Check sheet for the modelled part. Datum: model origin and axes. Units: mm. A direction names the side the tool comes from. Give positions to 0.01 mm unless a question says otherwise; leave off trailing zeros. Loops run counter-clockwise (first coordinate to the right, second up) from the corner with the lowest first, then second, coordinate; pieces in that order, holes last. Notation, with made-up numbers: M 78.5,-11 L 104.5,-11 A8 cw 104.5,-4 Z; hole C -1.5,17.25 d3. An arc over 180 degrees is marked long. Write each question's results on one line, items separated by ' | '. Start each with the question number.
1. Sectioned sample at A-A on z = 3.25. Record the cut outline in (x, y).
2. Sectioned sample at C-C on y = -7.5. Record the cut outline in (x, z).
3. Sectioned sample at D-D on x = -13.5. Record the cut outline in (y, z), and give its area (3 significant figures).
4. Tool access check on faces 1 (the flat face through (-17.1, 4, 3)), 2 (the flat face through (-16.6, -6, 1)), 3 (the flat face through (19, 2.9, 13)). Record the directions out of +Z, -Z, +X, -X, +Y, -Y that give a thin tool (end or side, any length) a straight path to the whole face; none if there is none.
5. Material ranges on line 1 along Z through (x, y) = (10, -5.75); line 2 along X through (y, z) = (5, 20), recorded low to high.
6. Sectioned sample at B-B on z = 21.25. Record the cut outline in (x, y), and give its area (3 significant figures).
7. Draft check along Y on faces 4 (the flat face through (19.6, 5.8, 24)), 5 (the flat face through (-19.1, 6, 3)), 6 (the flat face through (-19, 2.9, 3)), 7 (the flat face through (19.1, 6, 13)). Enter one of: pulls with the +Y half, pulls with the -Y half, needs draft (parallel to the pull), parting line crosses it, or undercut.
8. Go/stop test with flat-tipped pins: pin 1 (0.6 mm diameter, centred on y = 7.5, z = 8.5, fed in from -X); pin 2 (1 mm diameter, centred on x = 18, z = 16, fed in from -Y); pin 3 (6 mm diameter, centred on x = -6.5, y = 6.5, fed in from +Z). Record where each tip stops, or that it passes through.
Autodesk Inventor part; units mm, degrees
ref_plane "YZ Plane" through (0, 0, 0) normal (1, 0, 0) x (0, 1, 0)
ref_plane "XZ Plane" through (0, 0, 0) normal (0, 1, 0) x (-1, 0, 0)
ref_plane "XY Plane" through (0, 0, 0) normal (0, 0, 1) x (1, 0, 0)
sketch "Sketch1" plane through (0, 0, 0) normal (0, 0, 1) x (1, 0, 0)
  line L0 (20.1, 8.7) -> (-20.1, 8.7)
  line L1 (-20.1, 8.7) -> (-20.1, -8.7)
  line L2 (-20.1, -8.7) -> (20.1, -8.7)
  line L3 (20.1, -8.7) -> (20.1, 8.7)
  line L4 (20.1, 8.7) -> (-20.1, -8.7) construction
  line L5 (-20.1, 8.7) -> (20.1, -8.7) construction
  line L6 (-20.1, -8.7) -> (-16.6, -8.7)
  line L7 (-16.6, -8.7) -> (-16.6, -3.5)
  line L8 (-16.6, -3.5) -> (-20.1, -3.5)
  line L9 (-20.1, -3.5) -> (-20.1, -8.7)
  point P0 (0, 0)
  point P1 (-16.6, -8.7)
  dimension "d0" = 40.2
  dimension "d1" = 17.4
  dimension "d3" = 5.2
  dimension "d20" = 36.7
extrude "Extrusion1" add sketch "Sketch1" along normal blind 2 contours L3 L2 L7 L8 L1 L0
sketch "Sketch2" plane through (0, 0, 2) normal (0, 0, 1) x (1, 0, 0)
  line L0 (-20.1, 8.7) -> (-20.1, -3.5)
  line L1 (-20.1, 8.7) -> (-17.1, 8.7)
  line L2 (-17.1, 8.7) -> (-17.1, 2.9)
  line L3 (-17.1, 2.9) -> (-20.1, 2.9)
  line L4 (-20.1, 2.9) -> (-20.1, 8.7)
  line L5 (20.1, -8.7) -> (20.1, 8.7)
  line L6 (20.1, 8.7) -> (17.1, 8.7)
  line L7 (17.1, 8.7) -> (17.1, 2.9)
  line L8 (17.1, 2.9) -> (20.1, 2.9)
  line L9 (20.1, 2.9) -> (20.1, 8.7)
  line L10 (-20.1, 2.9) -> (-17.1, 2.9)
  line L11 (-17.1, 2.9) -> (-17.1, 4.9)
  line L12 (-17.1, 4.9) -> (-20.1, 4.9)
  line L13 (-20.1, 4.9) -> (-20.1, 2.9)
  line L14 (-20.1, 8.7) -> (-17.1, 8.7)
  line L15 (-17.1, 8.7) -> (-17.1, 6.7)
  line L16 (-17.1, 6.7) -> (-20.1, 6.7)
  line L17 (-20.1, 6.7) -> (-20.1, 8.7)
  line L18 (-20.1, 6.7) -> (-19.1, 6.7)
  line L19 (-19.1, 6.7) -> (-19.1, 4.9)
  line L20 (-19.1, 4.9) -> (-20.1, 4.9)
  line L21 (-20.1, 4.9) -> (-20.1, 6.7)
  line L22 (20.1, 8.7) -> (17.1, 8.7)
  line L23 (17.1, 8.7) -> (17.1, 6.7)
  line L24 (17.1, 6.7) -> (20.1, 6.7)
  line L25 (20.1, 6.7) -> (20.1, 8.7)
  line L26 (17.1, 2.9) -> (20.1, 2.9)
  line L27 (20.1, 2.9) -> (20.1, 4.9)
  line L28 (20.1, 4.9) -> (17.1, 4.9)
  line L29 (17.1, 4.9) -> (17.1, 2.9)
  line L30 (20.1, 4.9) -> (19.1, 4.9)
  line L31 (19.1, 4.9) -> (19.1, 6.7)
  line L32 (19.1, 6.7) -> (20.1, 6.7)
  line L33 (20.1, 6.7) -> (20.1, 4.9)
  point P0 (0, 0)
  dimension "d6" = 3
  dimension "d7" = 5.8
  dimension "d8" = 3
  dimension "d9" = 5.8
  dimension "d10" = 2
  dimension "d11" = 2
  dimension "d12" = 1
  dimension "d13" = 2
  dimension "d14" = 2
  dimension "d15" = 1
extrude "Extrusion2" add sketch "Sketch2" along normal blind 3 contours L1 L2 L16 L0 | L16 L19 L12 L0 | L12 L2 L3 L0 | L8 L7 L28 L5 | L28 L31 L24 L5 | L24 L7 L6 L5
sketch "Sketch3" plane through (0, 0, 5) normal (0, 0, 1) x (1, 0, 0)
  line L0 (17.1, 4.9) -> (17.1, 2.9)
  line L1 (17.1, 2.9) -> (20.1, 2.9)
  line L2 (20.1, 2.9) -> (20.1, 8.7)
  line L3 (20.1, 8.7) -> (17.1, 8.7)
  line L4 (17.1, 8.7) -> (17.1, 6.7)
  line L5 (17.1, 6.7) -> (19.1, 6.7)
  line L6 (19.1, 6.7) -> (19.1, 4.9)
  line L7 (19.1, 4.9) -> (17.1, 4.9)
  line L8 (19.1, 6.7) -> (20.1, 6.7)
  point P0 (0, 0)
extrude "Extrusion3" add sketch "Sketch3" along normal blind 19
properties part number "clip_zs042-command" material "PC/ABS Plastic"
Output values:
1) outline: M -20.1,2.9 L -17.1,2.9 L -17.1,4.9 L -19.1,4.9 L -19.1,6.7 L -17.1,6.7 L -17.1,8.7 L -20.1,8.7 Z; M 17.1,2.9 L 20.1,2.9 L 20.1,8.7 L 17.1,8.7 L 17.1,6.7 L 19.1,6.7 L 19.1,4.9 L 17.1,4.9 Z
2) outline: M -16.6,0 L 20.1,0 L 20.1,2 L -16.6,2 Z
3) outline: M -8.7,0 L 8.7,0 L 8.7,2 L -8.7,2 Z | area: 34.8 mm2
4) face 1: +Z, +Y, -Y | face 2: +Z, -Z, -X, -Y | face 3: +Z, +X, -X, -Y
5) line 1: 0 to 2 | line 2: 19.1 to 20.1
6) outline: M 17.1,2.9 L 20.1,2.9 L 20.1,8.7 L 17.1,8.7 L 17.1,6.7 L 19.1,6.7 L 19.1,4.9 L 17.1,4.9 Z | area: 13.8 mm2
7) face 4: needs draft | face 5: undercut | face 6: pulls with the -Y half | face 7: undercut
8) pin 1: x = 17.1 | pin 2: y = 2.9 | pin 3: z = 2
